```python
from build123d import *

# Parameters (mm, degrees)
SKETCH1_W           = 300
SKETCH1_H           = 40
SKETCH1_R           = 1.5
BOSS_EXTRUDE1_DEPTH = 1.5
CUT_EXTRUDE1_DEPTH  = 152.35719342


with BuildPart() as part:
    # Sketch1 → Boss-Extrude1 (new, symmetric)
    with BuildSketch(Plane(origin=(0, 0, 0), x_dir=(1, 0, 0), z_dir=(0, 1, 0))):
        Rectangle(SKETCH1_W, SKETCH1_H)
        with Locations(Location((-15.25, 15.25, 0), (0, 0, 270))):
            Circle(SKETCH1_R, mode=Mode.SUBTRACT)
        with Locations(Location((15.25, 15.25, 0), (0, 0, 270))):
            Circle(SKETCH1_R, mode=Mode.SUBTRACT)
        with Locations(Location((15.25, -15.25, 0), (0, 0, 270))):
            Circle(SKETCH1_R, mode=Mode.SUBTRACT)
        with Locations(Location((-15.25, -15.25, 0), (0, 0, 270))):
            Circle(SKETCH1_R, mode=Mode.SUBTRACT)
    extrude(amount=BOSS_EXTRUDE1_DEPTH, both=True)

    # Sketch2 → Cut-Extrude1 (cut, through all)
    with BuildSketch(Plane.XZ.offset(1.5)):
        Polygon((-150, 20), (-150, 10), (-45, 10), (-25, 20), align=None)
        Polygon((150, 20), (25, 20), (45, 10), (150, 10), align=None)
        Polygon((150, -20), (150, -10), (45, -10), (25, -20), align=None)
        Polygon((-150, -20), (-25, -20), (-45, -10), (-150, -10), align=None)
    extrude(amount=-CUT_EXTRUDE1_DEPTH, mode=Mode.SUBTRACT)


solid = part.part
```
Part model, mm, in its own coordinate system. Round coordinates to 2 decimals unless told otherwise and drop trailing zeros. Loops run counter-clockwise (first coordinate to the right, second up) from the corner with the lowest first, then second, coordinate; pieces in that order, holes last. Notation, with made-up numbers: (86, -39.75) -> (125, -39.75) arc R25 cw to (125, -7.75) -> close; hole circle Ø2 at (36, 80). An arc over 180 degrees is marked (long way). Use a Markdown table: item, result.
1) Cut at C-C, the plane x = 42. List the corners of the cut face in (y, z), and give its area (3 significant figures).
The answers:
| item | result |
|---|---|
| outline | (-1.5, -11.5) -> (1.5, -11.5) -> (1.5, 11.5) -> (-1.5, 11.5) -> close |
| area | 69.0 mm2 |
2) Probe line 1 (X direction, y = -0.75, z = 15); line 2 (X direction, y = 0.4, z = 14); line 3 (Z direction, x = -130, y = -0.4). List the from-to ranges inside material, lowest first. Write a range as [from, to].
The answers:
| item | result |
|---|---|
| line 1 | x = [-35, -16.73], [-13.77, 13.77], [16.73, 35] |
| line 2 | x = [-37, -16.08], [-14.42, 14.42], [16.08, 37] |
| line 3 | z = [-10, 10] |
3) Cut at A-A, the plane y = 0.3. List the corners of the cut face in (x, z), and give its area (3 significant figures).
The answers:
| item | result |
|---|---|
| outline | (-150, -10) -> (-45, -10) -> (-25, -20) -> (25, -20) -> (45, -10) -> (150, -10) -> (150, 10) -> (45, 10) -> (25, 20) -> (-25, 20) -> (-45, 10) -> (-150, 10) -> close; hole circle Ø3 at (-15.25, -15.25); hole circle Ø3 at (-15.25, 15.25); hole circle Ø3 at (15.25, -15.25); hole circle Ø3 at (15.25, 15.25) |
| area | 7,370 mm2 |
4) Drop flat-ended pins along their axis: pin 1 Ø1.5 at (y, z) = (0.5, -12) entering from -X; pin 2 Ø1.5 at (x, y) = (-103, 0.5) entering from -Z; pin 3 Ø0.9 at (x, y) = (-74, -0.5) entering from +Z. Give the stop position or say it passes through.
The answers:
| item | result |
|---|---|
| pin 1 | stops at x = -42.5 |
| pin 2 | stops at z = -10 |
| pin 3 | stops at z = 10 |
5) Cut at B-B, the plane x = -66.5. List the corners of the cut face in (y, z), and give its area (3 significant figures).
The answers:
| item | result |
|---|---|
| outline | (-1.5, -10) -> (1.5, -10) -> (1.5, 10) -> (-1.5, 10) -> close |
| area | 60.0 mm2 |
